Verification items for the finished model (mm, model axes). A direction names the side the tool comes from. Coordinates: 2 decimals unless noted, no trailing zeros. Order: outer loops, then holes, each group sorted by start corner. A loop starts at its lowest first (then second) coordinate and runs counter-clockwise, first axis right, second up. Notation, with made-up numbers: M 83,73 L 117,73 A13 ccw 117,92 Z; hole C 2.25,75.5 d10. An arc over 180 degrees is marked long. Write item = value, one per line.
```python
from build123d import *

# Parameters (mm, degrees)
SKETCH1_W                  = 609.6
SKETCH1_H                  = 609.6
BOSS_EXTRUDE1_DEPTH        = 6.35
SKETCH2_W                  = 609.6
SKETCH2_H                  = 222.25
BOSS_EXTRUDE2_DEPTH        = 25.4
F_5_3_5_3_DIAMETER_HOLE1_D = 5.3


with BuildPart() as part:
    # Sketch1 → Boss-Extrude1 (new body)
    with BuildSketch(Plane(origin=(0, 0, 0), x_dir=(1, 0, 0), z_dir=(0, 1, 0))):
        with Locations((304.8, 304.8)):
            Rectangle(SKETCH1_W, SKETCH1_H)
    extrude(amount=BOSS_EXTRUDE1_DEPTH)

    # Sketch2 → Boss-Extrude2 (add)
    with BuildSketch(Plane(origin=(0, 6.35, 0), x_dir=(1, 0, 0), z_dir=(0, 1, 0))):
        with Locations((304.8, 498.475)):
            Rectangle(SKETCH2_W, SKETCH2_H)
    extrude(amount=BOSS_EXTRUDE2_DEPTH)

    # Ø5.3 (5.3) Diameter Hole1 (through all)
    with Locations(Plane(origin=(0, 6.35, 0), x_dir=(1, 0, 0), z_dir=(0, 1, 0))):
        with Locations((25.4, 368.3), (50.8, 368.3), (76.2, 368.3), (25.4, 342.9), (25.4, 317.5), (25.4, 69.85), (25.4, 44.45), (25.4, 19.05), (50.8, 19.05), (76.2, 19.05), (304.8, 19.05), (25.4, 193.675), (304.8, 368.3), (584.2, 193.675), (533.4, 368.3), (558.8, 368.3), (584.2, 368.3), (584.2, 342.9), (584.2, 317.5), (584.2, 69.85), (584.2, 44.45), (584.2, 19.05), (558.8, 19.05), (533.4, 19.05)):
            Hole(F_5_3_5_3_DIAMETER_HOLE1_D / 2)


solid = part.part
```
Item 1: Sectioned sample at A-A, the plane x = 477. Enter the section's corners in (y, z), then the cut area to 3 significant figures.
Report:
outline = M 0,-609.6 L 31.75,-609.6 L 31.75,-387.35 L 6.35,-387.35 L 6.35,0 L 0,0 Z
area = 9,520 mm^2
Item 2: Sectioned sample at C-C, the plane y = 17. Enter the section's corners in (x, z).
Report:
outline = M 0,-609.6 L 609.6,-609.6 L 609.6,-387.35 L 0,-387.35 Z
Item 3: Scan lines: L1, parallel to Z at x = 76, y = 2; L2, parallel to X at y = 4, z = -44; L3, parallel to Y at x = 304, z = -162. Record each from-to range of solid material in increasing order. Write a range as from..to.
Report:
L1 = -609.6..-370.94, -365.66..-21.69, -16.41..0
L2 = 0..22.79, 28.01..581.59, 586.81..609.6
L3 = 0..6.35
Item 4: Tool access check on faces 1 (the flat face through (301, 19, -387.35)), 2 (the flat face through (301, 31.75, -500)). Record the directions out of +Z, -Z, +X, -X, +Y, -Y that give a thin tool (end or side, any length) a straight path to the whole face; none if there is none.
Report:
face_1 = +Z, +X, -X, +Y
face_2 = +Z, -Z, +X, -X, +Y
Item 5: Gauge pin test, flat ends, axial feed: pin 1 (5 mm diameter, centred on y = 5, z = -418, fed in from -X); pin 2 (5 mm diameter, centred on x = 25.4, z = -19.05, fed in from +Y); pin 3 (7 mm diameter, centred on x = 533.4, z = -368.3, fed in from +Y); pin 4 (1.5 mm diameter, centred on x = 359, y = 19, fed in from +Z). Record the tip position at first contact, or that the pin passes through.
Report:
pin_1 = 0
pin_2 = through
pin_3 = 6.35
pin_4 = -387.35
Item 6: Sectioned sample at B-B, the plane z = -250. Enter the section's corners in (x, y).
Report:
outline = M 0,0 L 609.6,0 L 609.6,6.35 L 0,6.35 Z
